Design review of the part built by this model. Coordinates are the model's own, in mm. Coordinates: 2 decimals unless noted, no trailing zeros. Order: outer loops, then holes, each group sorted by start corner. A loop starts at its lowest first (then second) coordinate and runs counter-clockwise, first axis right, second up. Notation, with made-up numbers: M 66,-8 L 121,-8 A33 cw 121,22 Z; hole C 11,17.5 d10. An arc over 180 degrees is marked long. Answer in a Markdown table with one row per item.
from build123d import *

# Parameters (mm, degrees)
BOSS_EXTRUDE1_DEPTH = 1.3335
CUT_EXTRUDE1_START  = -3.667
SKETCH2_R           = 1.7145
CUT_EXTRUDE1_DEPTH  = 4.667
CIRPATTERN1_COUNT   = 5


with BuildPart() as part:
    # Sketch1 → Boss-Extrude1 (new body, symmetric)
    with BuildSketch(Plane(origin=(0, 0, 0), x_dir=(1, 0, 0), z_dir=(0, 1, 0))):
        Polygon((0, 0), (-63.5, -87.40025195), (0, -87.40025195), (63.5, -87.40025195), align=None)
    boss_extrude1 = extrude(amount=BOSS_EXTRUDE1_DEPTH, both=True)

    # Sketch2 → Cut-Extrude1 (cut)
    with BuildSketch(Plane.XZ.offset(1.3335).offset(CUT_EXTRUDE1_START)):
        with Locations((-44.45, 82.63775195)):
            Circle(SKETCH2_R)
        with Locations((0, 82.63775195)):
            Circle(SKETCH2_R)
        with Locations((44.45, 82.63775195)):
            Circle(SKETCH2_R)
    cut_extrude1 = extrude(amount=CUT_EXTRUDE1_DEPTH, mode=Mode.SUBTRACT)

    # CirPattern1: Boss-Extrude1, Cut-Extrude1 ×5 about axis
    cirpattern1_axis = Axis((0, 0, 0), (0, 1, 0))
    for i in range(1, CIRPATTERN1_COUNT):
        add(boss_extrude1.rotate(cirpattern1_axis, i * 360 / CIRPATTERN1_COUNT))
        add(cut_extrude1.rotate(cirpattern1_axis, i * 360 / CIRPATTERN1_COUNT), mode=Mode.SUBTRACT)


solid = part.part
(1) Insertion check: pin 1 Ø2 at (x, z) = (78.59, 25.54) entering from -Y; pin 2 Ø1 at (x, y) = (-74.5, -0.5) entering from -Z; pin 3 Ø1.5 at (y, z) = (0, -70.5) entering from +X. Each pin has a flat end and moves straight along its axis. Give the tip position at first contact, or say it passes through.
Return value:
| item | result |
|---|---|
| pin 1 | passes through |
| pin 2 | stops at z = -54.27 |
| pin 3 | stops at x = 52.69 |
(2) Add section B-B, the plane z = 36. Give the boundary of the cut face in (x, y), and give its area (3 significant figures).
Return value:
| item | result |
|---|---|
| outline | M -80.2,-1.33 L 80.2,-1.33 L 80.2,1.33 L -80.2,1.33 Z |
| area | 428 mm2 |
(3) For line 1 along X through (y, z) = (-1.1, 69); line 2 along X through (y, z) = (-0.05, -15.5); line 3 along X through (y, z) = (-0.7, 55), list the stretches that pass through material, from the lowest coordinate up. Write a range as from..to.
Return value:
| item | result |
|---|---|
| line 1 | x = -69.48..-66.09, -63.62..63.62, 66.09..69.48 |
| line 2 | x = -96.93..-93.52, -91.14..91.14, 93.52..96.93 |
| line 3 | x = -74.03..74.03 |
(4) Add section C-C, the plane x = -57. Give the boundary of the cut face in (y, z).
Return value:
| item | result |
|---|---|
| outline | M -1.33,-66.62 L 1.33,-66.62 L 1.33,87.4 L -1.33,87.4 Z |
(5) Add section A-A, the plane y = 0.4. Give the number of separate pieces and of enclosed holes in the cut face, and give its area (3 significant figures).
Return value:
| item | result |
|---|---|
| separate pieces | 1 |
| enclosed holes | 15 |
| area | 27,600 mm2 |
